Read the model definition and answer for the solid it produces. Units are mm, in the model's axes. Face numbers are marked on the shaded views. A direction names the side the tool comes from. Coordinates: 2 decimals unless noted, no trailing zeros. Loops run counter-clockwise (first coordinate to the right, second up) from the corner with the lowest first, then second, coordinate; pieces in that order, holes last. Notation, with made-up numbers: (82, 8) -> (94, 8) arc R18 cw to (94, 38) -> close; hole circle Ø1 at (61, 60.25). An arc over 180 degrees is marked (long way). Answer as a JSON object with one key per item and string values. Group by question number.
Q1. The part is cut by section B-B on y = 6.5. Write down the section's boundary in (x, z), and give its area (3 significant figures).
Q2. The part is cut by section D-D on y = 1.75. Write down the section's boundary in (x, z), and give its area (3 significant figures).
Q3. For the marked faces 1 and 2, determine the directions among +Z, -Z, +X, -X, +Y, -Y from which every point of the face is accessible in a straight line to the end or side of a thin tool.
Q4. The part is cut by section A-A on z = -34.4. Write down the section's boundary in (x, y), and give its area (3 significant figures).
Q5. Each of these flat-tipped pins is pushed along its axis until it touches: P1, Ø3, axis at x = 34.4, z = -5.6, coming from the -Y side; P2, Ø3, axis at x = 34, z = -8, coming from the +Y side; P3, Ø1.2, axis at x = 20.5, y = 7, coming from the -Z side; P4, Ø1.2, axis at x = 19.5, y = 7, coming from the +Z side. Where does it stop, or does it pass through?
Q6. The part is cut by section C-C on x = 5.6. Write down the section's boundary in (y, z).
Q7. Straight lines are drawn through the part: line 1 along X through (y, z) = (1.35, -34.4); line 2 along Y through (x, z) = (29.5, -36). For each, find the intervals that lie inside material, in ascending order. Write a range as [from, to].
Q8. Determine the mould class of the marked faces 3, 4 and 5 for opening direction Z: released by +Z, released by -Z, zero draft, split by the parting line, or undercut.
from build123d import *

# Parameters (mm, degrees)
SKETCH1_W           = 40
SKETCH1_H           = 40
SKETCH1_R           = 1.6
BOSS_EXTRUDE1_DEPTH = 6
SKETCH2_R           = 7.5
SKETCH2_R_2         = 5.25
BOSS_EXTRUDE2_DEPTH = 1.5
CUT_EXTRUDE1_DEPTH  = 21.5


with BuildPart() as part:
    # Sketch1 → Boss-Extrude1 (new body)
    with BuildSketch(Plane(origin=(0, 0, 0), x_dir=(1, 0, 0), z_dir=(0, 1, 0))):
        with Locations((20, 20)):
            Rectangle(SKETCH1_W, SKETCH1_H)
        with Locations(Location((5.6, 34.4, 0), (0, 0, 270))):
            Circle(SKETCH1_R, mode=Mode.SUBTRACT)
        with Locations(Location((5.6, 5.6, 0), (0, 0, 270))):
            Circle(SKETCH1_R, mode=Mode.SUBTRACT)
        with Locations(Location((34.4, 34.4, 0), (0, 0, 270))):
            Circle(SKETCH1_R, mode=Mode.SUBTRACT)
        with Locations(Location((34.4, 5.6, 0), (0, 0, 270))):
            Circle(SKETCH1_R, mode=Mode.SUBTRACT)
    extrude(amount=BOSS_EXTRUDE1_DEPTH)

    # Sketch2 → Boss-Extrude2 (add)
    # profile 1 of 3: a face of its own
    with BuildSketch(Plane(origin=(0, 6, 0), x_dir=(1, 0, 0), z_dir=(0, 1, 0))):
        with Locations(Location((20, 20, 0), (0, 0, 90))):
            Circle(SKETCH2_R)
        with Locations((20, 20)):
            Circle(SKETCH2_R_2, mode=Mode.SUBTRACT)
    # profile 2 of 3: a face of its own
    with BuildSketch(Plane(origin=(0, 6, 0), x_dir=(1, 0, 0), z_dir=(0, 1, 0))):
        with BuildLine():
            ThreePointArc((23.082207001, 24.25), (20, 25.25), (16.917792999, 24.25))
            Line((16.917792999, 24.25), (23.082207001, 24.25))
        make_face()
    # profile 3 of 3: a face of its own
    with BuildSketch(Plane(origin=(0, 6, 0), x_dir=(1, 0, 0), z_dir=(0, 1, 0))):
        with BuildLine():
            Line((23.082207001, 15.75), (16.917792999, 15.75))
            ThreePointArc((16.917792999, 15.75), (20, 14.75), (23.082207001, 15.75))
        make_face()
    extrude(amount=BOSS_EXTRUDE2_DEPTH)

    # Sketch4 → Cut-Extrude1 (cut)
    with BuildSketch(Plane(origin=(0, 6, 0), x_dir=(1, 0, 0), z_dir=(0, 1, 0))):
        with BuildLine():
            Line((16, 20.5), (18, 20.5))
            ThreePointArc((18, 20.5), (18.5, 20), (18, 19.5))
            Line((18, 19.5), (16, 19.5))
            ThreePointArc((16, 19.5), (15.5, 20), (16, 20.5))
        make_face()
        with BuildLine():
            Line((24, 19.5), (22, 19.5))
            ThreePointArc((22, 19.5), (21.5, 20), (22, 20.5))
            Line((22, 20.5), (24, 20.5))
            ThreePointArc((24, 20.5), (24.5, 20), (24, 19.5))
        make_face()
    extrude(amount=-CUT_EXTRUDE1_DEPTH, mode=Mode.SUBTRACT)


solid = part.part
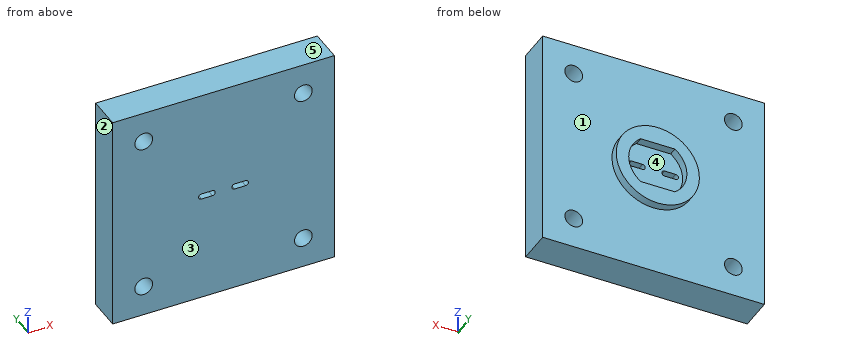
Final values:
{
 "1": {"outline": "circle Ø15 at (20, -20); hole (16.92, -24.25) -> (23.08, -24.25) arc R5.25 ccw to (23.08, -15.75) -> (16.92, -15.75) arc R5.25 ccw to start", "area": "98.5 mm2"},
 "2": {"outline": "(0, -40) -> (40, -40) -> (40, 0) -> (0, 0) -> close; hole circle Ø3.2 at (5.6, -34.4); hole circle Ø3.2 at (5.6, -5.6); hole (16, -20.5) -> (18, -20.5) arc R0.5 ccw to (18, -19.5) -> (16, -19.5) arc R0.5 ccw to start; hole (22, -20.5) -> (24, -20.5) arc R0.5 ccw to (24, -19.5) -> (22, -19.5) arc R0.5 ccw to start; hole circle Ø3.2 at (34.4, -34.4); hole circle Ø3.2 at (34.4, -5.6)", "area": "1,560 mm2"},
 "3": {"face 1": "+Y", "face 2": "+Z, -Z, -X, +Y, -Y"},
 "4": {"outline": "(0, 0) -> (4, 0) -> (4, 6) -> (0, 6) -> close; (7.2, 0) -> (32.8, 0) -> (32.8, 6) -> (7.2, 6) -> close; (36, 0) -> (40, 0) -> (40, 6) -> (36, 6) -> close", "area": "202 mm2"},
 "5": {"P1": "passes through", "P2": "stops at y = 6", "P3": "stops at z = -27.5", "P4": "stops at z = -12.5"},
 "6": {"outline": "(0, -40) -> (6, -40) -> (6, -36) -> (0, -36) -> close; (0, -32.8) -> (6, -32.8) -> (6, -7.2) -> (0, -7.2) -> close; (0, -4) -> (6, -4) -> (6, 0) -> (0, 0) -> close"},
 "7": {"line 1": "x = [0, 4], [7.2, 32.8], [36, 40]", "line 2": "y = [0, 6]"},
 "8": {"face 3": "zero draft", "face 4": "undercut", "face 5": "released by +Z"}
}
